Input: part model. Units: mm. Frame: model coordinates. A direction names the side the tool comes from. Coordinates: 2 decimals unless noted, no trailing zeros. Order: outer loops, then holes, each group sorted by start corner. A loop starts at its lowest first (then second) coordinate and runs counter-clockwise, first axis right, second up. Notation, with made-up numbers: M -28,24 L -19,24 A10 ccw -19,39 Z; hole C 87.25,48 d5. An arc over 180 degrees is marked long. Answer in a Markdown table with one row per item.
from build123d import *

# Parameters (mm, degrees)
BOSS_EXTRUDE3_DEPTH = 3
SKETCH13_R          = 4
SKETCH13_R_2        = 1.7859375
BOSS_EXTRUDE4_DEPTH = 5
SKETCH14_R          = 4
CUT_EXTRUDE8_DEPTH  = 1.5
SKETCH15_R          = 1.875
CUT_EXTRUDE9_DEPTH  = 4.0000001


with BuildPart() as part:
    # Sketch11 → Boss-Extrude3 (new body)
    with BuildSketch(Plane(origin=(0, 0, 0), x_dir=(1, 0, 0), z_dir=(0, 1, 0))):
        with BuildLine():
            Line((37.748131547, 6.010178191), (37.748131547, -17.989821809))
            ThreePointArc((37.748131547, -17.989821809), (36.576558672, -20.818248934), (33.748131547, -21.989821809))
            add(Edge.make_bspline(
                [(-36.251868453, -21.989821809), (-30.327598806, -21.989821809), (-19.243874055, -24.873158899), (-7.077839403, -30.012200103), (4.574088551, -30.012200103), (16.743326023, -24.873158899), (27.816510145, -21.989821809), (33.748131547, -21.989821809)],
                knots=[0, 0, 0, 0, 0.248449553, 0.474844955, 0.525155045, 0.751550447, 1, 1, 1, 1], degree=3))
            ThreePointArc((-36.251868453, -21.989821809), (-39.080295577, -20.818248934), (-40.251868453, -17.989821809))
            Line((-40.251868453, -17.989821809), (-40.251868453, 6.010178191))
            ThreePointArc((-40.251868453, 6.010178191), (-39.080295577, 8.838605316), (-36.251868453, 10.010178191))
            add(Edge.make_bspline(
                [(-36.251868453, 10.010178191), (-30.320247051, 10.010178191), (-19.247062928, 12.893515281), (-7.077825456, 18.032556484), (4.574102497, 18.032556484), (16.74013715, 12.893515281), (27.8238619, 10.010178191), (33.748131547, 10.010178191)],
                knots=[0, 0, 0, 0, 0.248449553, 0.474844955, 0.525155045, 0.751550447, 1, 1, 1, 1], degree=3))
            ThreePointArc((33.748131547, 10.010178191), (36.576558672, 8.838605316), (37.748131547, 6.010178191))
        make_face()
    extrude(amount=-BOSS_EXTRUDE3_DEPTH)

    # Sketch13 → Boss-Extrude4 (add)
    with BuildSketch(Plane(origin=(0, 0, 0), x_dir=(1, 0, 0), z_dir=(0, 1, 0))):
        with Locations(Location((-36.251868453, -17.989821809, 0), (0, 0, 270))):  # turned: the seam where the file's is
            Circle(SKETCH13_R)
        with Locations(Location((-36.251868453, -17.989821809, 0), (0, 0, 270))):  # turned: the seam where the file's is
            Circle(SKETCH13_R_2, mode=Mode.SUBTRACT)
        with Locations(Location((-36.251868453, 6.010178191, 0), (0, 0, 270))):  # turned: the seam where the file's is
            Circle(SKETCH13_R)
        with Locations(Location((-36.251868453, 6.010178191, 0), (0, 0, 270))):  # turned: the seam where the file's is
            Circle(SKETCH13_R_2, mode=Mode.SUBTRACT)
        with Locations(Location((33.748131547, 6.010178191, 0), (0, 0, 270))):  # turned: the seam where the file's is
            Circle(SKETCH13_R)
        with Locations(Location((33.748131547, 6.010178191, 0), (0, 0, 270))):  # turned: the seam where the file's is
            Circle(SKETCH13_R_2, mode=Mode.SUBTRACT)
        with Locations(Location((33.748131547, -17.989821809, 0), (0, 0, 270))):  # turned: the seam where the file's is
            Circle(SKETCH13_R)
        with Locations(Location((33.748131547, -17.989821809, 0), (0, 0, 270))):  # turned: the seam where the file's is
            Circle(SKETCH13_R_2, mode=Mode.SUBTRACT)
    extrude(amount=BOSS_EXTRUDE4_DEPTH)

    # Sketch14 → Cut-Extrude8 (cut)
    with BuildSketch(Plane(origin=(0, 0, 0), x_dir=(1, 0, 0), z_dir=(0, 1, 0))):
        with Locations(Location((-1.251868453, 13.010178191, 0), (0, 0, 270))):  # turned: the seam where the file's is
            Circle(SKETCH14_R)
        with Locations(Location((-1.251868453, -24.989821809, 0), (0, 0, 270))):  # turned: the seam where the file's is
            Circle(SKETCH14_R)
    extrude(amount=-CUT_EXTRUDE8_DEPTH, mode=Mode.SUBTRACT)

    # Sketch15 → Cut-Extrude9 (cut, through all)
    with BuildSketch(Plane(origin=(0, 0, 0), x_dir=(1, 0, 0), z_dir=(0, 1, 0))):
        with Locations(Location((-1.251868453, -24.989821809, 0), (0, 0, 270))):  # turned: the seam where the file's is
            Circle(SKETCH15_R)
        with Locations(Location((-1.251868453, 13.010178191, 0), (0, 0, 270))):  # turned: the seam where the file's is
            Circle(SKETCH15_R)
    extrude(amount=-CUT_EXTRUDE9_DEPTH, mode=Mode.SUBTRACT)


solid = part.part
1) Reachability of faces 1 (the face through (-37, 5, -4)), 2 (the face through (-0.05, -0.74, -9.195)) from +Z, -Z, +X, -X, +Y, -Y: full face, straight path, thin tool, end or side. Return the list, or none.
Resolved:
| item | result |
|---|---|
| face 1 | +Z, -Z, +X, -X, +Y |
| face 2 | +Y |
2) Material intervals for probe 1 along Y at (x, z) = (14, -10.5); probe 2 along Z at (x, y) = (33, -2.25); probe 3 along Z at (x, y) = (-19.5, -0.25) (3 decimals), sorted ascending.
Resolved:
| item | result |
|---|---|
| probe 1 | y = -3 to 0 |
| probe 2 | z = -10.02 to 22 |
| probe 3 | z = -13.255 to 25.235 |
3) Cut plane B-B, the plane z = 10. Output: boundary loops of the cut face in (x, y).
Resolved:
| item | result |
|---|---|
| outline | M -40.25,-3 L 37.75,-3 L 37.75,0 L -40.25,0 Z |
4) Mould query, pull axis X, two halves, no side actions, for faces 3 (the face through (33, 5, -4)), 4 (the face through (37.748, -1, 6)), 5 (the face through (-1.169, -2.24, -14.883)). Classes: +X half, -X half, draft (parallel to the pull), parting line (faces both ways), or undercut.
Resolved:
| item | result |
|---|---|
| face 3 | draft |
| face 4 | +X half |
| face 5 | undercut |
5) Cut plane C-C, the plane x = -2. State how many separate pieces and enclosed holes the cut face has, and give its area (3 significant figures).
Resolved:
| item | result |
|---|---|
| separate pieces | 3 |
| enclosed holes | 0 |
| area | 110 mm2 |
6) Cut plane A-A, the plane y = 2. Output: boundary loops of the cut face in (x, z), and give its area (3 significant figures).
Resolved:
| item | result |
|---|---|
| outline | C -36.25,-6.01 d8; C -36.25,17.99 d8; C 33.75,-6.01 d8; C 33.75,17.99 d8; hole C -36.25,-6.01 d3.57; hole C -36.25,17.99 d3.57; hole C 33.75,-6.01 d3.57; hole C 33.75,17.99 d3.57 |
| area | 161 mm2 |
7) Contact query for flat-ended pins moving along their axis: pin 1 (1.8 mm diameter, centred on x = 33, z = 18, fed in from +Y); pin 2 (3 mm diameter, centred on y = 0, z = 20, fed in from -X). Output: stop coordinate, or through.
Resolved:
| item | result |
|---|---|
| pin 1 | stops at y = 0 |
| pin 2 | stops at x = -40.22 |
